For this review, take the finished solid that the model builds, in its own axes (mm). Round coordinates to 2 decimals unless told otherwise and drop trailing zeros. Loops run counter-clockwise (first coordinate to the right, second up) from the corner with the lowest first, then second, coordinate; pieces in that order, holes last.
1) Take a section at C-C (x = 17). State the section outline as (y, z) points.
2) Insertion check: pin 1 (2 mm diameter, centred on y = -26.5, z = 1, fed in from -X); pin 2 (3 mm diameter, centred on x = 48, z = 3, fed in from +Y); pin 3 (1.5 mm diameter, centred on x = 12, y = 20.5, fed in from -Z); pin 4 (1.9 mm diameter, centred on y = 5.5, z = 2.5, fed in from +X). Each pin has a flat end and moves straight along its axis. Give the tip position at first contact, or say it passes through.
3) Take a section at B-B (y = 9). State the section outline as (x, z) points, then the cut area to 3 significant figures.
4) Wall thickness on L1, parallel to X at y = 30.5, z = 1; L2, parallel to Y at x = -46, z = 3.25; L3, parallel to Y at x = 21.5, z = 3.25: over which ranges is each line inside the solid? List them lowest first.
5) Take a section at A-A (y = 36.5). State the section outline as (x, z) points, then the cut area to 3 significant figures.
```python
from build123d import *

# Parameters (mm, degrees)
SKETCH2_W           = 101.6
SKETCH2_H           = 101.6
BOSS_EXTRUDE3_DEPTH = 6.35
SKETCH3_W           = 6.35
SKETCH3_H           = 25.4
SKETCH3_W_2         = 31.1
SKETCH3_W_3         = 31.100053481
SKETCH3_W_4         = 6.34997326
SKETCH3_H_2         = 25.400000079
SKETCH3_H_3         = 25.399999921
SKETCH3_W_5         = 31.100486926
SKETCH3_H_4         = 12.7
CUT_EXTRUDE1_DEPTH  = 73.122135992


with BuildPart() as part:
    # Sketch2 → Boss-Extrude3 (new body)
    with BuildSketch(Plane.XY):
        Rectangle(SKETCH2_W, SKETCH2_H)
    extrude(amount=BOSS_EXTRUDE3_DEPTH)

    # Sketch3 → Cut-Extrude1 (cut, through all)
    with BuildSketch(Plane.XY.offset(6.35)):
        with Locations((-47.625, 38.1)):
            Rectangle(SKETCH3_W, SKETCH3_H)
        with Locations((-22.55, 38.1)):
            Rectangle(SKETCH3_W_2, SKETCH3_H)
        with Locations((-47.625, 0)):
            Rectangle(SKETCH3_W, SKETCH3_H)
        with Locations((22.550026741, 38.1)):
            Rectangle(SKETCH3_W_3, SKETCH3_H)
        with Locations((-47.625, -38.1)):
            Rectangle(SKETCH3_W, SKETCH3_H)
        with Locations((47.62501337, 38.1)):
            Rectangle(SKETCH3_W_4, SKETCH3_H)
        with Locations((47.62501337, -3.9e-08)):
            Rectangle(SKETCH3_W_4, SKETCH3_H_2)
        Polygon((-7.000486295, -38.1), (-38.1, -38.1), (-38.1, -50.8), (-6.999486151, -50.8), align=None)
        with Locations((47.62501337, -38.10000004)):
            Rectangle(SKETCH3_W_4, SKETCH3_H_3)
        with Locations((22.549757168, -44.45)):
            Rectangle(SKETCH3_W_5, SKETCH3_H_4)
    extrude(amount=-CUT_EXTRUDE1_DEPTH, mode=Mode.SUBTRACT)


solid = part.part
```
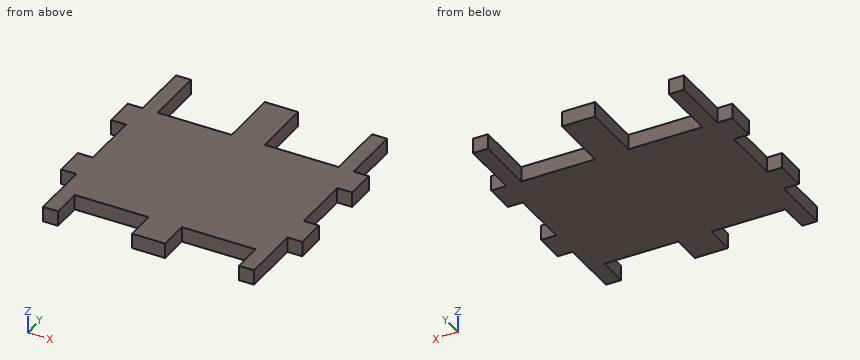
Response:
1. outline: (-38.1, 0) - (25.4, 0) - (25.4, 6.35) - (-38.1, 6.35) - close
2. pin 1: stops at x = -44.45
2. pin 2: stops at y = 25.4
2. pin 3: stops at z = 0
2. pin 4: stops at x = 44.45
3. outline: (-44.45, 0) - (44.45, 0) - (44.45, 6.35) - (-44.45, 6.35) - close
3. area: 565 mm2
4. L1: x = -44.45 to -38.1, -7 to 7, 38.1 to 44.45
4. L2: y = -25.4 to -12.7, 12.7 to 25.4
4. L3: y = -38.1 to 25.4
5. outline: (-44.45, 0) - (-38.1, 0) - (-38.1, 6.35) - (-44.45, 6.35) - close; (-7, 0) - (7, 0) - (7, 6.35) - (-7, 6.35) - close; (38.1, 0) - (44.45, 0) - (44.45, 6.35) - (38.1, 6.35) - close
5. area: 170 mm2
